Autodesk Inventor part; units mm, degrees
ref_plane "YZ Plane" through (0, 0, 0) normal (1, 0, 0) x (0, 1, 0)
ref_plane "XZ Plane" through (0, 0, 0) normal (0, 1, 0) x (-1, 0, 0)
ref_plane "XY Plane" through (0, 0, 0) normal (0, 0, 1) x (1, 0, 0)
sketch "Sketch1" plane through (0, 0, 0) normal (0, 1, 0) x (-1, 0, 0)
  line L0 (-1.5, 0) -> (-3, 0)
  line L1 (-3, 0) -> (-3, -2)
  line L2 (-3, -3) -> (-3, -6)
  line L3 (-3, -6) -> (-2, -6)
  line L4 (0, -7.2) -> (0, 1.2)
  line L5 (-3, -3) -> (-2.5, -3)
  line L6 (-2.5, -3) -> (-2.5, -2)
  line L7 (-2.5, -2) -> (-3, -2)
  line L8 (-2, -6) -> (-2, 0)
  point P0 (0, 0)
  dimension "d1" = 2
  dimension "d4" = 3
  dimension "d9" = 0.5
revolve "Revolution1" add sketch "Sketch1" angle 360 about axis through (0, 0, -10) along (0, 0, 1)
properties part number "M4-HEATINSERT"
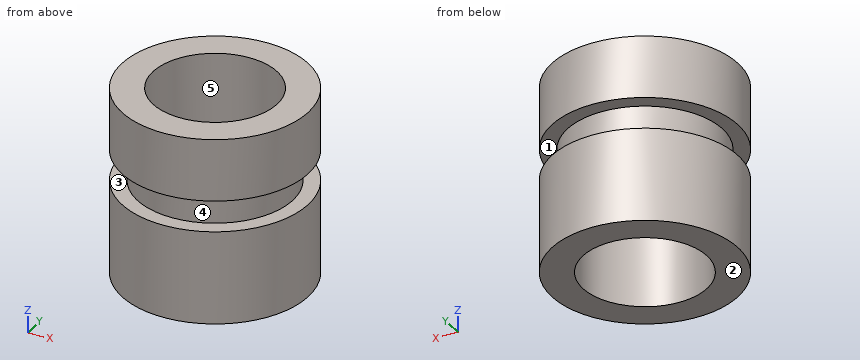
Source: CAD feature listing. Evaluate the final solid. Frame: model axes, mm. Face numbers are marked on the shaded views. A direction names the side the tool comes from. Give positions to 0.01 mm unless a question says otherwise; leave off trailing zeros. Loops run counter-clockwise (first coordinate to the right, second up) from the corner with the lowest first, then second, coordinate; pieces in that order, holes last. Notation, with made-up numbers: (-32, 55) -> (-22, 55) arc R29 cw to (-22, 77) -> close; hole circle Ø5 at (14.5, 29.5). An arc over 180 degrees is marked (long way). Use a Markdown table: item, result. Add a question column.
1) Section query C-C, the plane z = -1.9. Return the cut outline in (x, y).
2) Section query D-D, the plane x = 2.2. Return the cut outline in (y, z).
3) Pull-direction query (X, two-part tool) for the marked faces 3, 4 and 5; classes: +X half, -X half, draft (parallel to the pull), parting line (faces both ways), or undercut.
4) Reachability of the marked faces 1 and 2 from +Z, -Z, +X, -X, +Y, -Y: full face, straight path, thin tool, end or side. Return the list, or none.
5) First-contact query: pin 1 (1 mm diameter, centred on x = -1, z = -4.5, fed in from -Y); pin 2 (3 mm diameter, centred on x = 1, y = 1, fed in from -Z); pin 3 (1 mm diameter, centred on y = 1.5, z = -1.5, fed in from +X). Flat tips, straight axial feed; report the tip coordinate or a pass-through.
6) Line query: line 1 along Y through (x, z) = (0, -2.1); line 2 along Y through (x, z) = (0, -1.3). Output: solid intervals per line, ascending. Write a range as [from, to].
7) Section query A-A, the plane y = 0. Return the cut outline in (x, z), then the cut area to 3 significant figures.
Numbers:
| question | item | result |
|---|---|---|
| 1 | outline | circle Ø6 at (0, 0); hole circle Ø4 at (0, 0) |
| 2 | outline | (-2.04, -6) -> (2.04, -6) -> (2.04, -3) -> (1.19, -3) -> (1.19, -2) -> (2.04, -2) -> (2.04, 0) -> (-2.04, 0) -> (-2.04, -2) -> (-1.19, -2) -> (-1.19, -3) -> (-2.04, -3) -> close |
| 3 | face 3 | draft |
| 3 | face 4 | parting line |
| 3 | face 5 | undercut |
| 4 | face 1 | none |
| 4 | face 2 | -Z, +X, -X, +Y, -Y |
| 5 | pin 1 | stops at y = -2.96 |
| 5 | pin 2 | stops at z = -6 |
| 5 | pin 3 | stops at x = 2.83 |
| 6 | line 1 | y = [-2.5, -2], [2, 2.5] |
| 6 | line 2 | y = [-3, -2], [2, 3] |
| 7 | outline | (-3, -6) -> (-2, -6) -> (-2, 0) -> (-3, 0) -> (-3, -2) -> (-2.5, -2) -> (-2.5, -3) -> (-3, -3) -> close; (2, -6) -> (3, -6) -> (3, -3) -> (2.5, -3) -> (2.5, -2) -> (3, -2) -> (3, 0) -> (2, 0) -> close |
| 7 | area | 11.0 mm2 |
